```python
from build123d import *

# Parameters (mm, degrees)
BOSS_EXTRUDE1_DEPTH     = 10
FILLET1_R               = 2
CUT_EXTRUDE1_DEPTH      = 24.772357897
CUT_EXTRUDE1_DEPTH_BACK = 24.772357897
SKETCH4_R               = 2.5


with BuildPart() as part:
    # Sketch3 → Boss-Extrude1 (new body)
    with BuildSketch(Plane.XY):
        with BuildLine():
            Line((-2.5, 4.205809256), (-2.5, 14.205809256))
            ThreePointArc((-2.5, 14.205809256), (0, 15.25), (2.5, 14.205809256))
            Line((2.5, 14.205809256), (2.5, 4.205809256))
            ThreePointArc((2.5, 4.205809256), (3.459684342, 3.459684342), (4.205809256, 2.5))
            Line((4.205809256, 2.5), (14.205809256, 2.5))
            ThreePointArc((14.205809256, 2.5), (15.25, 0), (14.205809256, -2.5))
            Line((14.205809256, -2.5), (4.205809256, -2.5))
            ThreePointArc((4.205809256, -2.5), (3.459684342, -3.459684342), (2.5, -4.205809256))
            Line((2.5, -4.205809256), (2.5, -14.205809256))
            ThreePointArc((2.5, -14.205809256), (0, -15.25), (-2.5, -14.205809256))
            Line((-2.5, -14.205809256), (-2.5, -4.205809256))
            ThreePointArc((-2.5, -4.205809256), (-3.459684342, -3.459684342), (-4.205809256, -2.5))
            Line((-4.205809256, -2.5), (-14.205809256, -2.5))
            ThreePointArc((-14.205809256, -2.5), (-15.25, 0), (-14.205809256, 2.5))
            Line((-14.205809256, 2.5), (-4.205809256, 2.5))
            ThreePointArc((-4.205809256, 2.5), (-3.459684342, 3.459684342), (-2.5, 4.205809256))
        make_face()
    extrude(amount=BOSS_EXTRUDE1_DEPTH)

    # Fillet1
    fillet1_edges = [part.edges().sort_by_distance(p)[0] for p in [
        (-2.5, 14.205809256, 5),
        (2.5, 14.205809256, 5),
        (14.205809256, 2.5, 5),
        (14.205809256, -2.5, 5),
        (2.5, -14.205809256, 5),
        (-2.5, -14.205809256, 5),
        (-14.205809256, -2.5, 5),
        (-14.205809256, 2.5, 5),
    ]]
    fillet(fillet1_edges, radius=FILLET1_R)

    # Sketch4 → Cut-Extrude1 (cut, two sides: drawn at the far end of the back side and taken through both)
    with BuildSketch(Plane.XY.offset(-CUT_EXTRUDE1_DEPTH_BACK)):
        Circle(SKETCH4_R)
    extrude(amount=CUT_EXTRUDE1_DEPTH + CUT_EXTRUDE1_DEPTH_BACK, mode=Mode.SUBTRACT)


solid = part.part
```
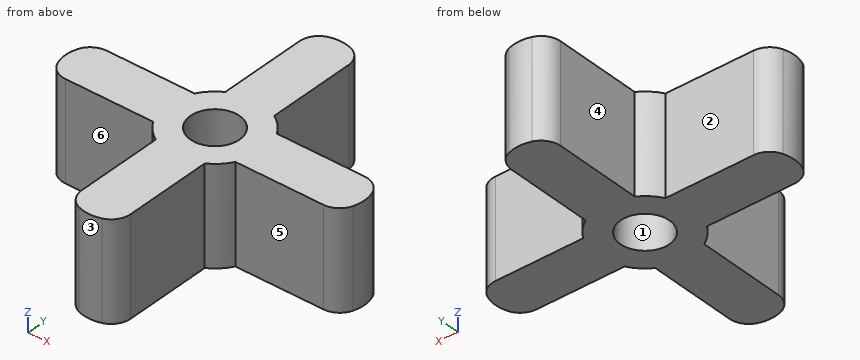
Model file for the job. Use its own axes, mm. Face numbers are marked on the shaded views. A direction names the side the tool comes from. Round coordinates to 2 decimals unless told otherwise and drop trailing zeros. Write each loop counter-clockwise with the first axis right and the second up, starting at its lowest first coordinate (ties: lowest second). Pieces come first, ordered by that corner, then holes. Notation, with made-up numbers: M 46,-20.75 L 50,-20.75 A14 ccw 50,-12.75 Z; hole C 16.5,70 d9. An arc over 180 degrees is marked long. Put each result on its own line as item: value.
Item 1: Flat gauge pins, fed straight in: P1, Ø4.5, axis at y = -8.5, z = 3, coming from the -X side; P2, Ø6, axis at x = 4.5, z = 5.5, coming from the +Y side; P3, Ø5, axis at y = 4, z = 8, coming from the -X side. Where does each tip first touch, or does it go through?
Responses:
P1: x = -2.5
P2: y = 14.9
P3: x = -14.9
Item 2: Probe L1, parallel to X at y = 0, z = 3.5; L2, parallel to X at y = -13, z = 4.25. List the from-to ranges inside material, lowest first. Write a range as from..to.
Responses:
L1: -15.25..-2.5, 2.5..15.25
L2: -2.5..2.5
Item 3: Mould opens along Y. For the marked faces 1, 2 and 3 say: +Y half, -Y half, draft (parallel to the pull), parting line (faces both ways), or undercut.
Responses:
face 1: undercut
face 2: +Y half
face 3: -Y half
Item 4: Cut at B-B (z = 0.75). List the corners of the cut face in (x, y).
Responses:
outline: M -15.05,-1.16 A2 ccw -13.17,-2.5 L -4.21,-2.5 A4.89 ccw -2.5,-4.21 L -2.5,-13.17 A2 ccw -1.16,-15.05 A3.51 ccw 1.16,-15.05 A2 ccw 2.5,-13.17 L 2.5,-4.21 A4.89 ccw 4.21,-2.5 L 13.17,-2.5 A2 ccw 15.05,-1.16 A3.51 ccw 15.05,1.16 A2 ccw 13.17,2.5 L 4.21,2.5 A4.89 ccw 2.5,4.21 L 2.5,13.17 A2 ccw 1.16,15.05 A3.51 ccw -1.16,15.05 A2 ccw -2.5,13.17 L -2.5,4.21 A4.89 ccw -4.21,2.5 L -13.17,2.5 A2 ccw -15.05,1.16 A3.51 ccw Z; hole C 0,0 d5
Item 5: Cut at A-A (y = 0). List the corners of the cut face in (x, z).
Responses:
outline: M -15.25,0 L -2.5,0 L -2.5,10 L -15.25,10 Z; M 2.5,0 L 15.25,0 L 15.25,10 L 2.5,10 Z
Item 6: Tool access for the marked faces 4, 5 and 6: list every direction of +Z, -Z, +X, -X, +Y, -Y with a clear straight run to the whole face (end or side of a thin tool).
Responses:
face 4: +Z, -Z, -X, +Y
face 5: +Z, -Z, +X, -Y
face 6: +Z, -Z, -X, -Y
Item 7: Cut at D-D (y = -10). List the corners of the cut face in (x, z).
Responses:
outline: M -2.5,0 L 2.5,0 L 2.5,10 L -2.5,10 Z
